from build123d import *

# Parameters (mm, degrees)
SKETCH1_R           = 254.5
SKETCH1_R_2         = 234.5
BOSS_EXTRUDE1_DEPTH = 5
SKETCH2_W           = 27.805822748
SKETCH2_H           = 60
CUT_EXTRUDE1_DEPTH  = 5
SKETCH3_R           = 2.5
CUT_EXTRUDE2_DEPTH  = 5
SKETCH4_R           = 1.5
CUT_EXTRUDE3_DEPTH  = 5
SKETCH5_W           = 651.212620435
SKETCH5_H           = 357.226439325
CUT_EXTRUDE4_DEPTH  = 10
CUT_EXTRUDE5_START  = -10
CUT_EXTRUDE5_DEPTH  = 10


with BuildPart() as part:
    # Sketch1 → Boss-Extrude1 (new body)
    with BuildSketch(Plane(origin=(0, 0, 0), x_dir=(1, 0, 0), z_dir=(0, 1, 0))):
        with Locations(Location((0, 0, 0), (0, 0, 270))):
            Circle(SKETCH1_R)
        with Locations(Location((0, 0, 0), (0, 0, 270))):
            Circle(SKETCH1_R_2, mode=Mode.SUBTRACT)
    extrude(amount=BOSS_EXTRUDE1_DEPTH)

    # Sketch2 → Cut-Extrude1 (cut)
    with BuildSketch(Plane(origin=(0, 5, 0), x_dir=(1, 0, 0), z_dir=(0, 1, 0))):
        with Locations((-240.597088626, 30)):
            Rectangle(SKETCH2_W, SKETCH2_H)
    cut_extrude1 = extrude(amount=-CUT_EXTRUDE1_DEPTH, mode=Mode.SUBTRACT)

    # Mirror1: Cut-Extrude1 across plane
    add(cut_extrude1.mirror(Plane.XY), mode=Mode.SUBTRACT)

    # Sketch3 → Cut-Extrude2 (cut)
    with BuildSketch(Plane(origin=(0, 5, 0), x_dir=(1, 0, 0), z_dir=(0, 1, 0))):
        with Locations(Location((242.5, 0, 0), (0, 0, 270))):
            Circle(SKETCH3_R)
        with Locations(Location((196.186621136, -142.537923681, 0), (0, 0, 270))):
            Circle(SKETCH3_R)
        with Locations(Location((74.936621136, -230.631205202, 0), (0, 0, 270))):
            Circle(SKETCH3_R)
        with Locations(Location((-74.936621136, -230.631205202, 0), (0, 0, 270))):
            Circle(SKETCH3_R)
        with Locations(Location((-196.186621136, -142.537923681, 0), (0, 0, 270))):
            Circle(SKETCH3_R)
        with Locations((-242.5, 0)):
            Circle(SKETCH3_R)
        with Locations(Location((-196.186621136, 142.537923681, 0), (0, 0, 270))):
            Circle(SKETCH3_R)
        with Locations(Location((-74.936621136, 230.631205202, 0), (0, 0, 270))):
            Circle(SKETCH3_R)
        with Locations(Location((74.936621136, 230.631205202, 0), (0, 0, 270))):
            Circle(SKETCH3_R)
        with Locations(Location((196.186621136, 142.537923681, 0), (0, 0, 270))):
            Circle(SKETCH3_R)
    extrude(amount=-CUT_EXTRUDE2_DEPTH, mode=Mode.SUBTRACT)

    # Sketch4 → Cut-Extrude3 (cut)
    with BuildSketch(Plane(origin=(0, 5, 0), x_dir=(1, 0, 0), z_dir=(0, 1, 0))):
        with Locations(Location((0, -242.5, 0), (0, 0, 270))):
            Circle(SKETCH4_R)
        with Locations(Location((-142.537923681, -196.186621136, 0), (0, 0, 270))):
            Circle(SKETCH4_R)
        with Locations(Location((-230.631205202, -74.936621136, 0), (0, 0, 270))):
            Circle(SKETCH4_R)
        with Locations(Location((-230.631205202, 74.936621136, 0), (0, 0, 270))):
            Circle(SKETCH4_R)
        with Locations(Location((-142.537923681, 196.186621136, 0), (0, 0, 270))):
            Circle(SKETCH4_R)
        with Locations(Location((0, 242.5, 0), (0, 0, 270))):
            Circle(SKETCH4_R)
        with Locations(Location((142.537923681, 196.186621136, 0), (0, 0, 270))):
            Circle(SKETCH4_R)
        with Locations(Location((230.631205202, 74.936621136, 0), (0, 0, 270))):
            Circle(SKETCH4_R)
        with Locations(Location((230.631205202, -74.936621136, 0), (0, 0, 270))):
            Circle(SKETCH4_R)
        with Locations(Location((142.537923681, -196.186621136, 0), (0, 0, 270))):
            Circle(SKETCH4_R)
    extrude(amount=-CUT_EXTRUDE3_DEPTH, mode=Mode.SUBTRACT)

    # Sketch5 → Cut-Extrude4 (cut)
    with BuildSketch(Plane(origin=(0, 5, 0), x_dir=(1, 0, 0), z_dir=(0, 1, 0))):
        with Locations((-71.106310217, -178.613219663)):
            Rectangle(SKETCH5_W, SKETCH5_H)
    extrude(amount=-CUT_EXTRUDE4_DEPTH, mode=Mode.SUBTRACT)

    # Sketch6 → Cut-Extrude5 (cut)
    with BuildSketch(Plane(origin=(0, 5, 0), x_dir=(1, 0, 0), z_dir=(0, 1, 0)).offset(CUT_EXTRUDE5_START)):
        with BuildLine():
            Line((254.5, 0), (0, 0))
            Line((0, 0), (-127.25, 220.403465263))
            ThreePointArc((-127.25, 220.403465263), (127.25, 220.403465263), (254.5, 0))
        make_face()
    extrude(amount=CUT_EXTRUDE5_DEPTH, mode=Mode.SUBTRACT)


solid = part.part
Geometry check sheet. Reference: the model listing, model coordinates, mm. Round coordinates to 2 decimals unless told otherwise and drop trailing zeros. Order: outer loops, then holes, each group sorted by start corner. A loop starts at its lowest first (then second) coordinate and runs counter-clockwise, first axis right, second up. Notation, with made-up numbers: M 69.5,42.25 L 77.5,42.25 A20 cw 77.5,63.25 Z; hole C 80.5,13.5 d11. An arc over 180 degrees is marked long. Answer in a Markdown table with one row per item. Add a question column.
Item 1: Material ranges on L1, parallel to X at y = 3.25, z = -143; L2, parallel to X at y = 3.85, z = -174; L3, parallel to X at y = 0.9, z = -209, recorded low to high. Write a range as [from, to].
Item 2: Sectioned sample at C-C, the plane x = -131. Enter the section's corners in (y, z).
Item 3: Sectioned sample at B-B, the plane y = 2.35. Enter the section's corners in (x, z), plus the area to 3 significant figures.
Item 4: Draft check along Z on faces 1 (the face through (-237, 3, -60)), 2 (the face through (-192, 0, -147)), 3 (the face through (-202.87, 2.46, -153.67)), 4 (the face through (-197.71, 2.54, -144.52)). Enter one of: released by +Z, released by -Z, zero draft, split by the parting line, or undercut.
Item 5: Depth check by flat-ended pin: pin 1 Ø1.5 at (y, z) = (3.5, -179.5) entering from -X. Enter the tip coordinate at first touch or a pass-through.
Item 6: Sectioned sample at D-D, the plane z = -180. Enter the section's corners in (x, y).
Item 7: Sectioned sample at A-A, the plane z = -143. Enter the section's corners in (x, y), plus the area to 3 significant figures.
Filled in:
| question | item | result |
|---|---|---|
| 1 | L1 | x = [-210.53, -198.64], [-193.73, -185.85] |
| 1 | L2 | x = [-185.73, -157.21] |
| 1 | L3 | x = [-145.22, -120.67] |
| 2 | outline | M 0,-218.2 L 5,-218.2 L 5,-194.5 L 0,-194.5 Z |
| 3 | outline | M -247.33,-60 A254.5 ccw -127.25,-220.4 L -117.25,-203.08 A234.5 cw -226.69,-60 Z; hole C -230.63,-74.94 d3; hole C -196.19,-142.54 d5; hole C -142.54,-196.19 d3 |
| 3 | area | 3,870 mm² |
| 4 | face 1 | released by +Z |
| 4 | face 2 | zero draft |
| 4 | face 3 | released by -Z |
| 4 | face 4 | undercut |
| 5 | pin 1 | stops at x = -181.16 |
| 6 | outline | M -179.92,0 L -150.3,0 L -150.3,5 L -179.92,5 Z |
| 7 | outline | M -210.53,0 L -198.64,0 L -198.64,5 L -210.53,5 Z; M -193.73,0 L -185.85,0 L -185.85,5 L -193.73,5 Z |
| 7 | area | 98.8 mm² |
